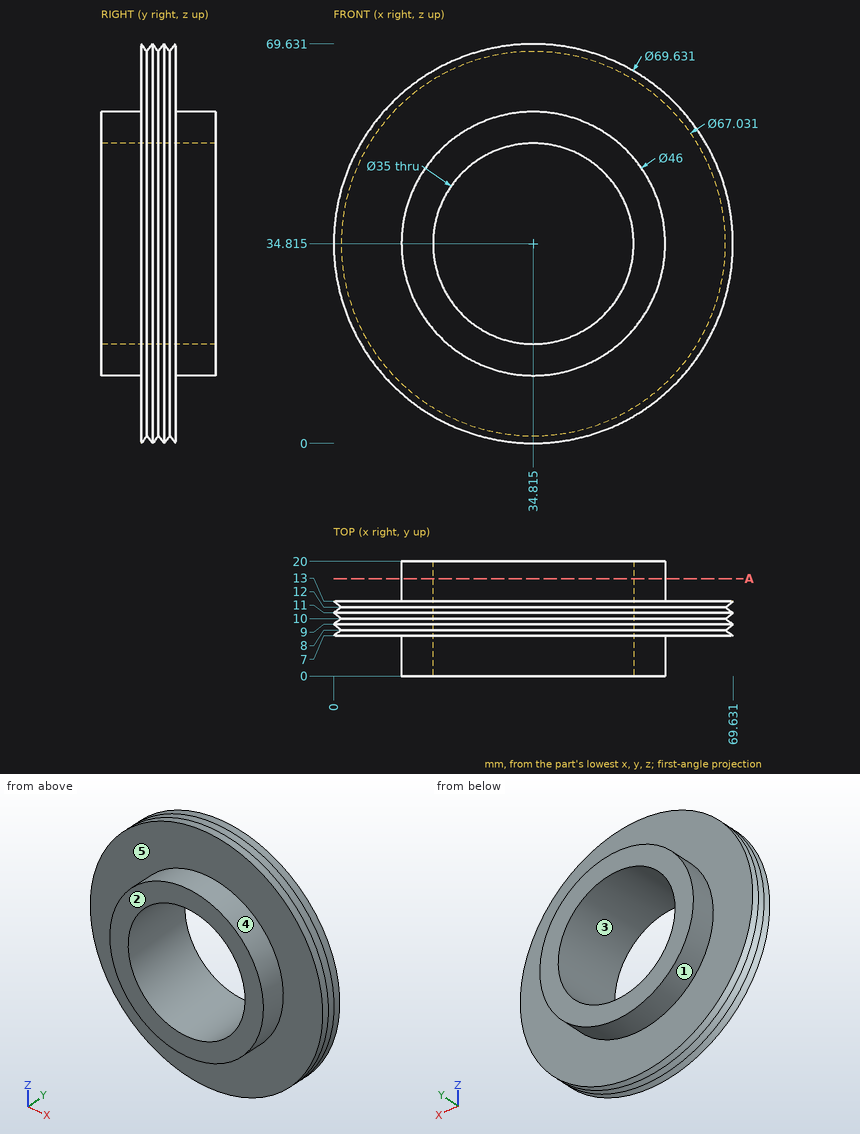
Verification items for this drawing (mm, ordinates from the low corner). A direction names the side the tool comes from. Coordinates: 2 decimals unless noted, no trailing zeros. Write each loop counter-clockwise with the first axis right and the second up, starting at its lowest first coordinate (ties: lowest second). Pieces come first, ordered by that corner, then holes. Notation, with made-up numbers: (23.5, 79.5) -> (53.5, 79.5) arc R20 cw to (53.5, 98.5) -> close; hole circle Ø9 at (19, 78.5). An arc over 180 degrees is marked (long way). One line per item, written item: value. Start each with the question number.
Q1. Mould release check, pull along X, two halves, no side actions. Record for the marked faces 3, 4 and 5: pulls with the +X half, pulls with the -X half, needs draft (parallel to the pull), parting line crosses it, or undercut.
Q2. Access from +Z, -Z, +X, -X, +Y, -Y to the whole of each face (thin tool, end or side, straight path). Record for the marked faces 1 and 2.
Q3. Go/stop test with flat-tipped pins: P1, Ø12, axis at x = 10.5, y = 4.5, coming from the +Z side; P2, Ø4, axis at y = 16.5, z = 61.5, coming from the -X side; P3, Ø3, axis at x = 56, z = 53.5, coming from the +Y side; P4, Ø1, axis at x = 19, y = 8.5, coming from the +Z side (1 decimal). Record where each tip stops, or that it passes through.
Q4. Cross-section at A-A on y = 17. Enter the section's corners in (x, z) (1 decimal), and give its area (3 significant figures).
Q5. Thickness scan on L1, parallel to Y at x = 56.5, z = 26.5; L2, parallel to X at y = 5, z = 38.5; L3, parallel to Z at x = 24.5, y = 6.25. Record the ranges inside material, lowest first. Write a range as from..to.
Checked values:
1. face 3: undercut
1. face 4: parting line crosses it
1. face 5: needs draft
2. face 1: +Y
2. face 2: +Z, -Z, +X, -X, -Y
3. P1: stops at z = 64.08
3. P2: passes through
3. P3: stops at y = 13
3. P4: stops at z = 65.9
4. outline: circle Ø46 at (34.8, 34.8); hole circle Ø35 at (34.8, 34.8)
4. area: 700 mm²
5. L1: y = 7..13
5. L2: x = 12.11..17.71, 51.92..57.52
5. L3: z = 14.26..20.68, 48.95..55.37
